```python
from build123d import *

# Parameters (mm, degrees)
BOSS_EXTRUDE1_DEPTH = 50
SKETCH3_R           = 1.6
CUT_EXTRUDE1_DEPTH  = 50
SKETCH4_R           = 5.1
CUT_EXTRUDE2_DEPTH  = 50


with BuildPart() as part:
    # Sketch2 → Boss-Extrude1 (new body)
    with BuildSketch(Plane.XY):
        Polygon((0, 0), (-82, 0), (-82, -28), (-79.5, -28), (-79.5, -2.5), (-2.5, -2.5), (-2.5, -60), (0, -60), align=None)
    extrude(amount=BOSS_EXTRUDE1_DEPTH)

    # Sketch3 → Cut-Extrude1 (cut)
    with BuildSketch(Plane.ZY.offset(82)):
        with Locations((12.5, -20)):
            Circle(SKETCH3_R)
        with Locations((37.5, -20)):
            Circle(SKETCH3_R)
    extrude(amount=-CUT_EXTRUDE1_DEPTH, mode=Mode.SUBTRACT)

    # Sketch4 → Cut-Extrude2 (cut)
    with BuildSketch(Plane(origin=(0, 0, 0), x_dir=(0, 0, -1), z_dir=(1, 0, 0))):
        with Locations((-35.2, -42.25)):
            Circle(SKETCH4_R)
    extrude(amount=-CUT_EXTRUDE2_DEPTH, mode=Mode.SUBTRACT)


solid = part.part
```
Can you work these out from the model? Positions are in its coordinate system, mm. A direction names the side the tool comes from. Round coordinates to 2 decimals unless told otherwise and drop trailing zeros. Loops run counter-clockwise (first coordinate to the right, second up) from the corner with the lowest first, then second, coordinate; pieces in that order, holes last. Notation, with made-up numbers: (68, 14) -> (124, 14) arc R21 cw to (124, 40) -> close; hole circle Ø6 at (-0.75, 37). An arc over 180 degrees is marked (long way). One line per item, written item: value. Start each with the question number.
1. If we section it at B-B, the plane y = -20: Write out the boundary of the cut face in (x, z).
2. If we mould it in two halves opening along Z, with no side actions, what happens to faces 1 (the flat face through (-32, -1, 50)), 2 (the flat face through (-42, -2.5, 25)), 3 (the cylindrical face through (-1.232, -40.718, 30.336))? For each: pulls with the +Z half, pulls with the -Z half, needs draft (parallel to the pull), parting line crosses it, or undercut.
3. For pin 1 (15 mm diameter, centred on x = -52, z = 34.5, fed in from -Y); pin 2 (3 mm diameter, centred on x = -81, z = 29.5, fed in from -Y); pin 3 (13.5 mm diameter, centred on y = -42.25, z = 35.2, fed in from +X); pin 4 (2.5 mm diameter, centred on y = -20, z = 37.5, fed in from -X), each with a flat end and sliding along its axis, tell me the tip position at first contact or that it passes through.
4. If we section it at D-D, the plane z = 37.5: Write out the boundary of the cut face in (x, y), then the cut area to 3 significant figures.
5. If I drill on probe 1 along X at (y, z) = (-3.5, 13.5); probe 2 along Y at (x, z) = (-18, 14.5), over which ranges is the centre line in solid material (lowest first)?
6. For faces 4 (the flat face through (-79.5, -15, 25)), 5 (the flat face through (0, -30, 25)), 6 (the cylindrical face through (-80.768, -18.414, 37.292)), 7 (the flat face through (-81, -28, 25)), which set-ups out of +Z, -Z, +X, -X, +Y, -Y let a thin tool reach every point of the face, with its end or its side?
7. If we section it at A-A, the plane z = 12.5: Write out the boundary of the cut face in (x, y), then the cut area to 4 significant figures.
8. If we section it at C-C, the plane y = -42.25: Write out the boundary of the cut face in (x, z), then the cut area to 3 significant figures.
Calculated:
1. outline: (-82, 0) -> (-79.5, 0) -> (-79.5, 10.9) -> (-82, 10.9) -> close; (-82, 14.1) -> (-79.5, 14.1) -> (-79.5, 35.9) -> (-82, 35.9) -> close; (-82, 39.1) -> (-79.5, 39.1) -> (-79.5, 50) -> (-82, 50) -> close; (-2.5, 0) -> (0, 0) -> (0, 50) -> (-2.5, 50) -> close
2. face 1: pulls with the +Z half
2. face 2: needs draft
2. face 3: undercut
3. pin 1: stops at y = -2.5
3. pin 2: stops at y = -28
3. pin 3: stops at x = 0
3. pin 4: stops at x = -2.5
4. outline: (-82, -28) -> (-79.5, -28) -> (-79.5, -21.6) -> (-82, -21.6) -> close; (-82, -18.4) -> (-79.5, -18.4) -> (-79.5, -2.5) -> (-2.5, -2.5) -> (-2.5, -37.7) -> (0, -37.7) -> (0, 0) -> (-82, 0) -> close; (-2.5, -60) -> (0, -60) -> (0, -46.8) -> (-2.5, -46.8) -> close
4. area: 382 mm²
5. probe 1: x = -82 to -79.5, -2.5 to 0
5. probe 2: y = -2.5 to 0
6. face 4: +Z, -Z, -Y
6. face 5: +Z, -Z, +X, +Y, -Y
6. face 6: -X
6. face 7: +Z, -Z, -X, -Y
7. outline: (-82, -28) -> (-79.5, -28) -> (-79.5, -21.6) -> (-82, -21.6) -> close; (-82, -18.4) -> (-79.5, -18.4) -> (-79.5, -2.5) -> (-2.5, -2.5) -> (-2.5, -60) -> (0, -60) -> (0, 0) -> (-82, 0) -> close
7. area: 404.5 mm²
8. outline: (-2.5, 0) -> (0, 0) -> (0, 30.1) -> (-2.5, 30.1) -> close; (-2.5, 40.3) -> (0, 40.3) -> (0, 50) -> (-2.5, 50) -> close
8. area: 99.5 mm²
